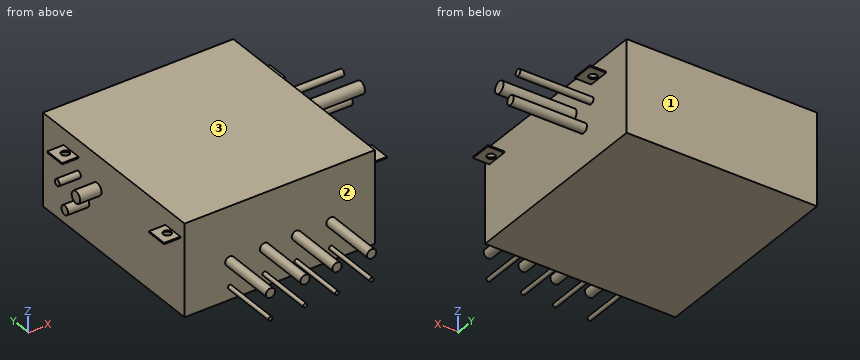
from build123d import *

# Parameters (mm, degrees)
F0_W          = 454.025
F0_H          = 219.075
F1_DEPTH      = 481.0125
F2_R          = 11.1125
F2_R_2        = 4.7625
F3_DEPTH      = 138.1125
F4_R          = 14.2875
F4_R_2        = 7.9375
F4_R_3        = 11.1125
F5_DEPTH      = 174.625
F5_DEPTH_BACK = 628.65
F7_W          = 38.89375
F7_H          = 50.8
F7_R          = 9.525
F8_DEPTH      = 3.175
F9_W          = 152.4
F9_H          = 219.075
F10_DEPTH     = 481.0135


with BuildPart() as f1:
    # F0 (on Front) → F1 (new body)
    with BuildSketch(Plane.XZ):
        with Locations((227.0125, 109.5375)):
            Rectangle(F0_W, F0_H)
    extrude(amount=-F1_DEPTH)

    # F2 (on Front) → F3 (join)
    with BuildSketch(Plane.XZ):
        with Locations((107.95, 90.4875)):
            Circle(F2_R)
        with Locations((107.95, 30.1625)):
            Circle(F2_R_2)
        with Locations((349.25, 90.4875)):
            Circle(F2_R)
        with Locations((349.25, 30.1625)):
            Circle(F2_R_2)
        with Locations((190.5, 90.4875)):
            Circle(F2_R)
        with Locations((266.7, 90.4875)):
            Circle(F2_R)
        with Locations((190.5, 30.1625)):
            Circle(F2_R_2)
        with Locations((266.7, 30.1625)):
            Circle(F2_R_2)
    extrude(amount=F3_DEPTH)

    # F4 (on face) → F5 (join, two sides)
    with BuildSketch(Plane.YZ.offset(454.025)) as f5_sk:
        with Locations((296.8625, 139.7)):
            Circle(F4_R)
        with Locations((360.3625, 139.7)):
            Circle(F4_R_2)
        with Locations((334.9625, 88.9)):
            Circle(F4_R_3)
    extrude(amount=F5_DEPTH)
    extrude(f5_sk.sketch, amount=-F5_DEPTH_BACK)

    # F7 (on offset) → F8 (join)
    with BuildSketch(Plane.XY.offset(180.975)):
        with Locations((-19.446875, 385.7625)):
            Rectangle(F7_W, F7_H)
        with Locations((-13.49375, 385.7625)):
            Circle(F7_R, mode=Mode.SUBTRACT)
        with Locations((-19.446875, 39.6875)):
            Rectangle(F7_W, F7_H)
        with Locations((-13.49375, 39.6875)):
            Circle(F7_R, mode=Mode.SUBTRACT)
        with Locations((473.471875, 385.7625)):
            Rectangle(F7_W, F7_H)
        with Locations((467.51875, 385.7625)):
            Circle(F7_R, mode=Mode.SUBTRACT)
        with Locations((473.471875, 39.6875)):
            Rectangle(F7_W, F7_H)
        with Locations((467.51875, 39.6875)):
            Circle(F7_R, mode=Mode.SUBTRACT)
    extrude(amount=-F8_DEPTH)

    # F9 (on face) → F10 (cut, through all)
    with BuildSketch(Plane.XZ):
        with Locations((-127, 109.5375)):
            Rectangle(F9_W, F9_H)
    extrude(amount=-F10_DEPTH, mode=Mode.SUBTRACT)


solid = f1.part
Geometry check sheet. Reference: the model listing, model coordinates, mm. Face numbers are marked on the shaded views. Round coordinates to 2 decimals unless told otherwise and drop trailing zeros. Write each loop counter-clockwise with the first axis right and the second up, starting at its lowest first coordinate (ties: lowest second). Pieces come first, ordered by that corner, then holes.
Item 1: Section check C-C (x = 404.5). Record the boundary of the cut face in (y, z) (1 decimal).
Determined:
outline: (0, 0) - (481, 0) - (481, 219.1) - (0, 219.1) - close
Item 2: Section check A-A (x = 585.5). Give the number of separate pieces and of enclosed holes in the cut face, plus the area to 3 significant figures.
Determined:
separate pieces: 3
enclosed holes: 0
area: 1,230 mm2
Item 3: Section check B-B (z = 15.5). Record the boundary of the cut face in (x, y) (1 decimal), plus the area to 3 significant figures.
Determined:
outline: (0, 0) - (454, 0) - (454, 481) - (0, 481) - close
area: 218,000 mm2
Item 4: Material ranges on line 1 along X through (y, z) = (125, 151.5) (3 decimals); line 2 along Y through (x, z) = (363.5, 97); line 3 along Z through (x, y) = (102, -53), recorded low to high.
Determined:
line 1: x = 0 to 454.025
line 2: y = 0 to 481.01
line 3: z = 81.1 to 99.87
Item 5: Go/stop test with flat-tipped pins: pin 1 Ø5 at (x, y) = (225, 403.5) entering from -Z; pin 2 Ø3 at (x, z) = (265.5, 64) entering from -Y; pin 3 Ø2.5 at (x, z) = (-11, 178.5) entering from +Y; pin 4 Ø2 at (y, z) = (343.5, 100) entering from +X (3 decimals). Record where each tip stops, or that it passes through.
Determined:
pin 1: stops at z = 0
pin 2: stops at y = 0
pin 3: stops at y = 411.16
pin 4: stops at x = 454.025
Item 6: Mould release check, pull along Y, two halves, no side actions. Record for the marked faces 1, 2 and 3: +Y half, -Y half, draft (parallel to the pull), parting line (faces both ways), or undercut.
Determined:
face 1: +Y half
face 2: -Y half
face 3: draft
